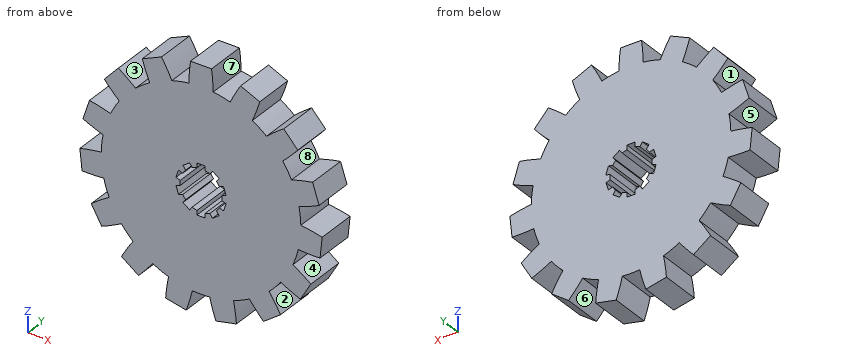
```python
from build123d import *

# Parameters (mm, degrees)
F1_DEPTH = 20


with BuildPart() as f1:
    # F0 (on Front) → F1 (new body)
    with BuildSketch(Plane.XZ):
        with BuildLine():
            ThreePointArc((-48.48151, 36.57166), (-44.837984, 32.512816), (-40.955282, 28.682135))
            ThreePointArc((-40.955282, 28.682135), (-43.30127, 25), (-45.317098, 21.127248))
            ThreePointArc((-45.317098, 21.127248), (-50.575917, 22.574425), (-55.912741, 23.700389))
            Line((-55.912741, 23.700389), (-59.165097, 13.690667))
            ThreePointArc((-59.165097, 13.690667), (-54.18569, 11.464684), (-49.080587, 9.54442))
            ThreePointArc((-49.080587, 9.54442), (-49.726095, 5.226423), (-49.992455, 0.868577))
            ThreePointArc((-49.992455, 0.868577), (-55.385245, 0.051685), (-60.718648, -1.090378))
            Line((-60.718648, -1.090378), (-59.618502, -11.557566))
            ThreePointArc((-59.618502, -11.557566), (-54.164198, -11.565795), (-48.719413, -11.243612))
            ThreePointArc((-48.719413, -11.243612), (-47.552826, -15.45085), (-46.023662, -19.540279))
            ThreePointArc((-46.023662, -19.540279), (-50.617961, -22.479992), (-55.025748, -25.692609))
            Line((-55.025748, -25.692609), (-49.763326, -34.807391))
            ThreePointArc((-49.763326, -34.807391), (-44.777225, -32.596444), (-39.934209, -30.087521))
            ThreePointArc((-39.934209, -30.087521), (-37.157241, -33.45653), (-34.09696, -36.570443))
            ThreePointArc((-34.09696, -36.570443), (-37.098372, -41.124674), (-39.818397, -45.852354))
            Line((-39.818397, -45.852354), (-31.303619, -52.038702))
            ThreePointArc((-31.303619, -52.038702), (-27.647862, -47.990872), (-24.244018, -43.729025))
            ThreePointArc((-24.244018, -43.729025), (-20.336832, -45.677273), (-16.274584, -47.277245))
            ThreePointArc((-16.274584, -47.277245), (-17.164137, -52.658526), (-17.726083, -58.083811))
            Line((-17.726083, -58.083811), (-7.431232, -60.272049))
            ThreePointArc((-7.431232, -60.272049), (-5.737933, -55.087241), (-4.361816, -49.809382))
            ThreePointArc((-4.361816, -49.809382), (0, -50), (4.361816, -49.809382))
            ThreePointArc((4.361816, -49.809382), (5.737933, -55.087241), (7.431232, -60.272049))
            Line((7.431232, -60.272049), (17.726083, -58.083811))
            ThreePointArc((17.726083, -58.083811), (17.164137, -52.658526), (16.274584, -47.277245))
            ThreePointArc((16.274584, -47.277245), (20.336832, -45.677273), (24.244018, -43.729025))
            ThreePointArc((24.244018, -43.729025), (27.647862, -47.990872), (31.303619, -52.038702))
            Line((31.303619, -52.038702), (39.818397, -45.852354))
            ThreePointArc((39.818397, -45.852354), (37.098372, -41.124674), (34.09696, -36.570443))
            ThreePointArc((34.09696, -36.570443), (37.157241, -33.45653), (39.934209, -30.087521))
            ThreePointArc((39.934209, -30.087521), (44.777225, -32.596444), (49.763326, -34.807391))
            Line((49.763326, -34.807391), (55.025748, -25.692609))
            ThreePointArc((55.025748, -25.692609), (50.617961, -22.479992), (46.023662, -19.540279))
            ThreePointArc((46.023662, -19.540279), (47.552826, -15.45085), (48.719413, -11.243612))
            ThreePointArc((48.719413, -11.243612), (54.164198, -11.565795), (59.618502, -11.557566))
            Line((59.618502, -11.557566), (60.718648, -1.090378))
            ThreePointArc((60.718648, -1.090378), (55.385245, 0.051685), (49.992455, 0.868577))
            ThreePointArc((49.992455, 0.868577), (49.726095, 5.226423), (49.080587, 9.54442))
            ThreePointArc((49.080587, 9.54442), (54.18569, 11.464684), (59.165097, 13.690667))
            Line((59.165097, 13.690667), (55.912741, 23.700389))
            ThreePointArc((55.912741, 23.700389), (50.575917, 22.574425), (45.317098, 21.127248))
            ThreePointArc((45.317098, 21.127248), (43.30127, 25), (40.955282, 28.682135))
            ThreePointArc((40.955282, 28.682135), (44.837984, 32.512816), (48.48151, 36.57166))
            Line((48.48151, 36.57166), (41.439014, 44.393143))
            ThreePointArc((41.439014, 44.393143), (37.021553, 41.193842), (32.806004, 37.732826))
            ThreePointArc((32.806004, 37.732826), (29.389263, 40.45085), (25.748437, 42.860448))
            ThreePointArc((25.748437, 42.860448), (27.737383, 47.939187), (29.415029, 53.12908))
            Line((29.415029, 53.12908), (19.800105, 57.40992))
            ThreePointArc((19.800105, 57.40992), (17.065827, 52.69047), (14.622453, 47.814055))
            ThreePointArc((14.622453, 47.814055), (10.395585, 48.90738), (6.089453, 49.6278))
            ThreePointArc((6.089453, 49.6278), (5.840736, 55.076436), (5.262422, 60.5))
            Line((5.262422, 60.5), (-5.262422, 60.5))
            ThreePointArc((-5.262422, 60.5), (-5.840736, 55.076436), (-6.089453, 49.6278))
            ThreePointArc((-6.089453, 49.6278), (-10.395585, 48.90738), (-14.622453, 47.814055))
            ThreePointArc((-14.622453, 47.814055), (-17.065827, 52.69047), (-19.800105, 57.40992))
            Line((-19.800105, 57.40992), (-29.415029, 53.12908))
            ThreePointArc((-29.415029, 53.12908), (-27.737383, 47.939187), (-25.748437, 42.860448))
            ThreePointArc((-25.748437, 42.860448), (-29.389263, 40.45085), (-32.806004, 37.732826))
            ThreePointArc((-32.806004, 37.732826), (-37.021553, 41.193842), (-41.439014, 44.393143))
            Line((-41.439014, 44.393143), (-48.48151, 36.57166))
        make_face()
        with BuildLine():
            ThreePointArc((-2.05, -10.297937), (-3.244678, -9.986093), (-4.39449, -9.536166))
            Line((-4.39449, -9.536166), (-5.71822, -11.358123))
            Line((-5.71822, -11.358123), (-9.03519, -8.948204))
            Line((-9.03519, -8.948204), (-7.71146, -7.126246))
            ThreePointArc((-7.71146, -7.126246), (-8.494678, -6.171745), (-9.160435, -5.131903))
            Line((-9.160435, -5.131903), (-11.302274, -5.827829))
            Line((-11.302274, -5.827829), (-12.569244, -1.928497))
            Line((-12.569244, -1.928497), (-10.427405, -1.232572))
            ThreePointArc((-10.427405, -1.232572), (-10.5, 0), (-10.427405, 1.232572))
            Line((-10.427405, 1.232572), (-12.569244, 1.928497))
            Line((-12.569244, 1.928497), (-11.302274, 5.827829))
            Line((-11.302274, 5.827829), (-9.160435, 5.131903))
            ThreePointArc((-9.160435, 5.131903), (-8.494678, 6.171745), (-7.71146, 7.126246))
            Line((-7.71146, 7.126246), (-9.03519, 8.948204))
            Line((-9.03519, 8.948204), (-5.71822, 11.358123))
            Line((-5.71822, 11.358123), (-4.39449, 9.536166))
            ThreePointArc((-4.39449, 9.536166), (-3.244678, 9.986093), (-2.05, 10.297937))
            Line((-2.05, 10.297937), (-2.05, 12.55))
            Line((-2.05, 12.55), (2.05, 12.55))
            Line((2.05, 12.55), (2.05, 10.297937))
            ThreePointArc((2.05, 10.297937), (3.244678, 9.986093), (4.39449, 9.536166))
            Line((4.39449, 9.536166), (5.71822, 11.358123))
            Line((5.71822, 11.358123), (9.03519, 8.948204))
            Line((9.03519, 8.948204), (7.71146, 7.126246))
            ThreePointArc((7.71146, 7.126246), (8.494678, 6.171745), (9.160435, 5.131903))
            Line((9.160435, 5.131903), (11.302274, 5.827829))
            Line((11.302274, 5.827829), (12.569244, 1.928497))
            Line((12.569244, 1.928497), (10.427405, 1.232572))
            ThreePointArc((10.427405, 1.232572), (10.5, 0), (10.427405, -1.232572))
            Line((10.427405, -1.232572), (12.569244, -1.928497))
            Line((12.569244, -1.928497), (11.302274, -5.827829))
            Line((11.302274, -5.827829), (9.160435, -5.131903))
            ThreePointArc((9.160435, -5.131903), (8.494678, -6.171745), (7.71146, -7.126246))
            Line((7.71146, -7.126246), (9.03519, -8.948204))
            Line((9.03519, -8.948204), (5.71822, -11.358123))
            Line((5.71822, -11.358123), (4.39449, -9.536166))
            ThreePointArc((4.39449, -9.536166), (3.244678, -9.986093), (2.05, -10.297937))
            Line((2.05, -10.297937), (2.05, -12.55))
            Line((2.05, -12.55), (-2.05, -12.55))
            Line((-2.05, -12.55), (-2.05, -10.297937))
        make_face(mode=Mode.SUBTRACT)
    extrude(amount=F1_DEPTH)


solid = f1.part
```
Check sheet for the modelled part. Datum: model origin and axes. Units: mm. Face numbers are marked on the shaded views. A direction names the side the tool comes from. Give positions to 0.01 mm unless a question says otherwise; leave off trailing zeros. Write each loop counter-clockwise with the first axis right and the second up, starting at its lowest first coordinate (ties: lowest second). Pieces come first, ordered by that corner, then holes.
Item 1: Cross-section at B-B (x = 52). Enter the section's corners in (y, z).
Item 2: Scan lines: L1, parallel to X at y = -1.5, z = 54.5; L2, parallel to X at y = -5.5, z = -10.5; L3, parallel to X at y = -1.25, z = -32.5. Record each from-to range of solid material in increasing order.
Item 3: Gauge pin test, flat ends, axial feed: pin 1 (5 mm diameter, centred on y = -6.5, z = -12, fed in from +X); pin 2 (0.7 mm diameter, centred on y = -7, z = -11.5, fed in from +X); pin 3 (12 mm diameter, centred on x = 11, y = -16.5, fed in from +Z); pin 4 (3 mm diameter, centred on x = 19, y = -12, fed in from +Z). Record the tip position at first contact, or that the pin passes through.
Item 4: Access from +Z, -Z, +X, -X, +Y, -Y to the whole of each face (thin tool, end or side, straight path). Record for the marked faces 4, 5, 6, 7 and 8.
Item 5: Draft check along X on the marked faces 1, 2 and 3. Enter one of: released by +X, released by -X, zero draft, split by the parting line, or undercut.
Item 6: Cross-section at A-A (z = -3.5). Enter the section's corners in (x, y), and give its area (3 significant figures).
Item 7: Cross-section at C-C (z = 40). Enter the section's corners in (x, y).
Item 8: Cross-section at D-D (z = 26). Enter the section's corners in (x, y).
Report:
1. outline: (-20, -30.93) - (0, -30.93) - (0, -23.44) - (-20, -23.44) - close; (-20, -11.48) - (0, -11.48) - (0, 0.6) - (-20, 0.6) - close; (-20, 10.6) - (0, 10.6) - (0, 22.91) - (-20, 22.91) - close
2. L1: x = -26.34 to -18.07, -5.88 to 5.88, 18.07 to 26.34
2. L2: x = -59.73 to -6.9, -5.09 to -2.05, 2.05 to 5.09, 6.9 to 59.73
2. L3: x = -51.1 to -44.58, -38 to 38, 44.58 to 51.1
3. pin 1: stops at x = 59.83
3. pin 2: stops at x = 59.66
3. pin 3: stops at z = 60.5
3. pin 4: stops at z = 57.41
4. face 4: +X, +Y, -Y
4. face 5: -X, +Y, -Y
4. face 6: -Z, +Y, -Y
4. face 7: +Z, +Y, -Y
4. face 8: +Y, -Y
5. face 1: released by -X
5. face 2: released by +X
5. face 3: undercut
6. outline: (-60.47, -20) - (-12.06, -20) - (-12.06, 0) - (-60.47, 0) - close; (12.06, -20) - (60.47, -20) - (60.47, 0) - (12.06, 0) - close
6. area: 1,940 mm2
7. outline: (-45.39, -20) - (-35.51, -20) - (-35.51, 0) - (-45.39, 0) - close; (-30, -20) - (30, -20) - (30, 0) - (-30, 0) - close; (35.51, -20) - (45.39, -20) - (45.39, 0) - (35.51, 0) - close
8. outline: (-42.71, -20) - (42.71, -20) - (42.71, 0) - (-42.71, 0) - close
